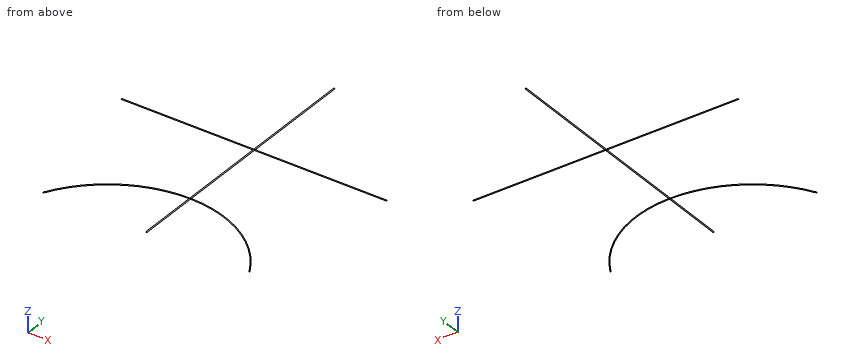
from build123d import *

# Parameters (mm, degrees)
SKETCH_R     = 1
PAD_DEPTH    = 450
SKETCH001_R  = 0.75
PAD001_DEPTH = 225
SKETCH002_R  = 0.75


with BuildPart() as part:
    # Sketch → Pad (new body)
    with BuildSketch(Plane.XZ):
        Circle(SKETCH_R)
    extrude(amount=-PAD_DEPTH)

    # Sketch001 → Pad001 (join, symmetric)
    with BuildSketch(Plane.YZ):
        with Locations((258, 0)):
            Circle(SKETCH001_R)
    extrude(amount=PAD001_DEPTH, both=True)

    # AdditivePipe: sweep along a path in Sketch003
    with BuildLine(Plane.XY) as additivepipe_path:
        ThreePointArc((175, 0), (102.041658, 76.736097), (0, 105))
        ThreePointArc((0, 105), (-102.041658, 76.736097), (-175, 0))
    # Sketch002 → AdditivePipe (sweep)
    with BuildSketch(Plane.YZ):
        with Locations((105, 0)):
            Circle(SKETCH002_R)
    sweep(path=additivepipe_path.line)


solid = part.part
The listing builds one solid part. Answer for the finished solid, in the listing's coordinates (mm). Coordinates: 2 decimals unless noted, no trailing zeros. Loops run counter-clockwise (first coordinate to the right, second up) from the corner with the lowest first, then second, coordinate; pieces in that order, holes last. Notation, with made-up numbers: M 55.25,54.25 L 79.25,54.25 A22 cw 79.25,71.25 Z; hole C 4,-8 d5. An arc over 180 degrees is marked long. Answer in a Markdown table with one row per item.
1) Given pin 1 (1 mm diameter, centred on x = -82.5, z = 0.5, fed in from +Y), flat-ended and moving along its own axis, determine where the tip first touches the part or whether it passes through.
Answers below:
| item | result |
|---|---|
| pin 1 | y = 258.75 |
2) Find the intervals of material crossed by probe 1 along X at (y, z) = (223, 0.55); probe 2 along X at (y, z) = (132, 0.3); probe 3 along Y at (x, z) = (-97.5, -0.35), in increasing order.
Answers below:
| item | result |
|---|---|
| probe 1 | -0.84 to 0.84 |
| probe 2 | -0.95 to 0.95 |
| probe 3 | 78.62 to 80.14, 257.34 to 258.66 |
3) Find section A-A (y = 321.5). Determine the outline of the cut face in (x, z).
Answers below:
| item | result |
|---|---|
| outline | C 0,0 d2 |
